```python
from build123d import *

# Parameters (mm, degrees)
SKETCH_1_W      = 56
SKETCH_1_H      = 85
SKETCH_1_R      = 1.5
EXTRUDE_1_DEPTH = 1.6
SKETCH_2_W      = 48.207961956
SKETCH_2_H      = 16.049260915
SKETCH_2_W_2    = 3.793795092
SKETCH_2_H_2    = 52.066933367
EXTRUDE_2_DEPTH = 10


with BuildPart() as part:
    # Sketch 1 → Extrude 1 (new body)
    with BuildSketch(Plane.XY):
        with Locations((14.816339797, 31.886417716)):
            Rectangle(SKETCH_1_W, SKETCH_1_H)
        with Locations((-9.683660203, 50.886417716)):
            Circle(SKETCH_1_R, mode=Mode.SUBTRACT)
        with Locations((39.316339797, 50.886417716)):
            Circle(SKETCH_1_R, mode=Mode.SUBTRACT)
        with Locations((-9.683660203, -7.113582284)):
            Circle(SKETCH_1_R, mode=Mode.SUBTRACT)
        with Locations((39.316339797, -7.113582284)):
            Circle(SKETCH_1_R, mode=Mode.SUBTRACT)
    extrude(amount=EXTRUDE_1_DEPTH)

    # Sketch 2 → Extrude 2 (add)
    with BuildSketch(Plane(origin=(0, 0, 0), x_dir=(-1, 0, 0), z_dir=(0, 0, -1))):
        with Locations((-15.098918569, 66.361787259)):
            Rectangle(SKETCH_2_W, SKETCH_2_H)
        with Locations((-37.306002001, 21.941048421)):
            Rectangle(SKETCH_2_W_2, SKETCH_2_H_2)
    extrude(amount=EXTRUDE_2_DEPTH)


solid = part.part
```
For this review, take the finished solid that the model builds, in its own axes (mm). A direction names the side the tool comes from. Round coordinates to 2 decimals unless told otherwise and drop trailing zeros. Order: outer loops, then holes, each group sorted by start corner. A loop starts at its lowest first (then second) coordinate and runs counter-clockwise, first axis right, second up. Notation, with made-up numbers: (2, 68) -> (11, 68) arc R28 cw to (11, 89) -> close; hole circle Ø8 at (66, 59). An arc over 180 degrees is marked (long way). Use a Markdown table: item, result.
Item 1: Machinability: for faces 4 (the flat face through (39.203, 22, -5)), 5 (the flat face through (-9.005, 66, -5)), 6 (the flat face through (35.409, 22, -5)), which of the approach directions +Z, -Z, +X, -X, +Y, -Y give a long, thin tool a straight path to every point of the face, cutting with its end or side? Answer none if there is none.
Resolved:
| item | result |
|---|---|
| face 4 | -Z, +X, +Y, -Y |
| face 5 | -Z, -X, +Y, -Y |
| face 6 | -Z, -X, -Y |
Item 2: For line 1 along X through (y, z) = (40, -8); line 2 along Z through (x, y) = (30.5, 26); line 3 along Y through (x, z) = (40.5, 1), list the stretches that pass through material, from the lowest coordinate up. Write a range as [from, to].
Resolved:
| item | result |
|---|---|
| line 1 | x = [35.41, 39.2] |
| line 2 | z = [0, 1.6] |
| line 3 | y = [-10.61, -8.03], [-6.19, 49.97], [51.81, 74.39] |
Item 3: Draft analysis for pull direction Y (two halves, no side actions). For faces 1 (the flat face through (14, 32, 1.6)), 2 (the flat face through (14, -10.614, 1)), 3 (the cylindrical face through (40.747, -6.663, 0.789)), state which applies: +Y half, -Y half, draft (parallel to the pull), parting line (faces both ways), or undercut.
Resolved:
| item | result |
|---|---|
| face 1 | draft |
| face 2 | -Y half |
| face 3 | undercut |
Item 4: For pin 1 (5 mm diameter, centred on y = 18, z = -7.5, fed in from -X); pin 2 (4 mm diameter, centred on x = 9.5, y = 12, fed in from -Z); pin 3 (3 mm diameter, centred on x = -2.5, z = -8.5, fed in from -Y); pin 4 (4 mm diameter, centred on x = -5, z = -0.5, fed in from -Y), all flat-tipped, find the tip position at first contact; note any pin that passes through.
Resolved:
| item | result |
|---|---|
| pin 1 | stops at x = 35.41 |
| pin 2 | stops at z = 0 |
| pin 3 | stops at y = 58.34 |
| pin 4 | stops at y = -10.61 |
Item 5: Take a section at A-A (z = -3). State the section outline as (x, y) points, plus the area to 3 significant figures.
Resolved:
| item | result |
|---|---|
| outline | (-9.01, 58.34) -> (39.2, 58.34) -> (39.2, 74.39) -> (-9.01, 74.39) -> close; (35.41, -4.09) -> (39.2, -4.09) -> (39.2, 47.97) -> (35.41, 47.97) -> close |
| area | 971 mm² |
Item 6: Take a section at B-B (x = 16). State the section outline as (y, z) points, plus the area to 3 significant figures.
Resolved:
| item | result |
|---|---|
| outline | (-10.61, 0) -> (58.34, 0) -> (58.34, -10) -> (74.39, -10) -> (74.39, 1.6) -> (-10.61, 1.6) -> close |
| area | 296 mm² |
Item 7: Take a section at C-C (y = 43). State the section outline as (x, z) points, plus the area to 3 significant figures.
Resolved:
| item | result |
|---|---|
| outline | (-13.18, 0) -> (35.41, 0) -> (35.41, -10) -> (39.2, -10) -> (39.2, 0) -> (42.82, 0) -> (42.82, 1.6) -> (-13.18, 1.6) -> close |
| area | 128 mm² |
